Solid Edge part; units mm, degrees
sketch "Sketch1" plane through (0, 0, 0) normal (0, -1, 0) x (1, 0, 0)
  line L0 (30, 0) -> (65, 15)
  line L1 (65, 15) -> (110, 15)
  line L2 (110, 15) -> (110, 20)
  line L3 (0, 20) -> (110, 20)
  line L4 (0, 20) -> (0, 15)
  line L5 (0, 15) -> (23, 15)
  line L6 (23, 15) -> (23, 8)
  line L7 (23, 8) -> (0, 8)
  line L8 (0, 8) -> (0, 0)
  line L9 (0, 0) -> (30, 0)
  dimension "D1" = 23
extrude "Protrusion1" add sketch "Sketch1" against normal blind 50
mirror "Mirror1" about plane through (0, 25, 4) normal (-1, 0, 0) of "Protrusion1"
sketch "Sketch2" plane through (0, 0, 26) normal (0, -1, 0) x (1, 0, 0)
  line L0 (30, -16.6796) -> (43.2525, -11)
  line L1 (43.2525, -11) -> (30, -11)
  line L2 (30, -11) -> (30, -16.6796)
extrude "Cutout1" cut sketch "Sketch2" against normal through all
sketch "Sketch3" plane through (0, 25, 0) normal (0, 0, -1) x (1, 0, 0)
  circle A0 centre (-16, 21) radius 1.75
  circle A1 centre (16, 21) radius 1.75
  circle A2 centre (16, -21) radius 1.75
  circle A3 centre (-16, -21) radius 1.75
extrude "Cutout2" cut sketch "Sketch3" against normal up to next
sketch "Sketch4" plane through (0, 25, 8) normal (0, 0, 1) x (1, 0, 0)
  circle A0 centre (-16, -21) radius 3.75
  circle A1 centre (16, -21) radius 3.75
  circle A2 centre (-16, 21) radius 3.75
  circle A3 centre (16, 21) radius 3.75
extrude "Extrusionsausschnitt_4" cut sketch "Sketch4" against normal blind 4
mirror "Mirror2" about plane through (0, 0, 0) normal (1, 0, 0) of "Cutout1"
sketch "Sketch5" plane through (0, 25, 20) normal (0, 0, 1) x (1, 0, 0)
  line L0 (110, -40) -> (-110, -40)
  line L1 (-110, -40) -> (-110, 40)
  line L2 (-110, 40) -> (110, 40)
  line L3 (110, 40) -> (110, -40)
  dimension "D1" = 110
extrude "Protrusion2" add sketch "Sketch5" against normal up to vertex (5 mm away)
sketch "Sketch6" plane through (0, 25, 20) normal (0, 0, 1) x (1, 0, 0)
  circle A0 centre (-97.5, -32.5) radius 2.25
  circle A1 centre (-47.5, 32.5) radius 2.25
  circle A2 centre (-47.5, -32.5) radius 2.25
  circle A3 centre (47.5, 32.5) radius 2.25
  circle A4 centre (47.5, -32.5) radius 2.25
  circle A5 centre (97.5, -32.5) radius 2.25
  circle A6 centre (97.5, 32.5) radius 2.25
  circle A7 centre (-97.5, 32.5) radius 2.25
extrude "Cutout3" cut sketch "Sketch6" against normal up to next
chamfer "Fase_2" distance 0.5 angle 45 8 edges at (-95.25, -7.5, 15) (-95.25, 57.5, 15) (-45.25, 57.5, 15) (49.75, 57.5, 15) (99.75, 57.5, 15) (99.75, -7.5, 15) (49.75, -7.5, 15) (-45.25, -7.5, 15)
hole "Hole_1" at (-16, 46, 20) direction (0, 0, -1) diameter 10 end up to next
hole "Hole1" at (-16, 4, 20) direction (0, 0, -1) diameter 10 end up to next
hole "Hole2" at (16, 4, 20) direction (0, 0, -1) diameter 10 end up to next
hole "Hole3" at (16, 46, 20) direction (0, 0, -1) diameter 10 end up to next
properties material "Nylon, allgemein"
Input: part model. Units: mm. Frame: model coordinates. A direction names the side the tool comes from. Give positions to 0.01 mm unless a question says otherwise; leave off trailing zeros. Order: outer loops, then holes, each group sorted by start corner. A loop starts at its lowest first (then second) coordinate and runs counter-clockwise, first axis right, second up. Notation, with made-up numbers: (-16, -22.5) -> (25, -22.5) arc R13 cw to (25, -3.5) -> close; hole circle Ø5 at (80.5, 69.5). An arc over 180 degrees is marked (long way). Use one line per item in the form item = value.
1) First-contact query: pin 1 Ø4 at (x, y) = (-97.5, 57.5) entering from +Z; pin 2 Ø4.5 at (x, z) = (18.5, 10) entering from +Y; pin 3 Ø1 at (y, z) = (26, 13.5) entering from +X; pin 4 Ø2 at (y, z) = (37.5, 10.5) entering from +X. Flat tips, straight axial feed; report the tip coordinate or a pass-through.
Response values:
pin_1 = through
pin_2 = 50
pin_3 = 62.67
pin_4 = 56.83
2) Line query: probe 1 along Y at (x, z) = (16, 2.7); probe 2 along Y at (x, z) = (-47.5, 18); probe 3 along X at (y, z) = (49, 15.75). Output: solid intervals per line, ascending.
Response values:
probe_1 = 0 to 2.25, 5.75 to 44.25, 47.75 to 50
probe_2 = -15 to -9.75, -5.25 to 55.25, 59.75 to 65
probe_3 = -110 to -20, -12 to 12, 20 to 110
3) Section C-C, the plane y = 20. Return loops of the section in (x, z), and give its area (3 significant figures).
Response values:
outline = (-110, 15) -> (-65, 15) -> (-30, 0) -> (30, 0) -> (65, 15) -> (110, 15) -> (110, 20) -> (-110, 20) -> close; hole (-43.25, 15) -> (-30, 9.32) -> (-30, 15) -> close; hole (-23, 8) -> (23, 8) -> (23, 15) -> (-23, 15) -> close; hole (30, 9.32) -> (43.25, 15) -> (30, 15) -> close
area = 2,130 mm^2
4) Reachability of faces 1 (the flat face through (0.9, 50, 7.6)), 2 (the flat face through (0, 25, 8)), 3 (the cylindrical face through (-19, 50, 18)) from +Z, -Z, +X, -X, +Y, -Y: full face, straight path, thin tool, end or side. Return the list, or none.
Response values:
face_1 = -Z, +X, -X, +Y
face_2 = +Y, -Y
face_3 = +Z
5) Mould query, pull axis X, two halves, no side actions, for faces 4 (the flat face through (2, -15, 18)), 5 (the flat face through (30, 25, 12)). Classes: pulls with the +X half, pulls with the -X half, needs draft (parallel to the pull), parting line crosses it, or undercut.
Response values:
face_4 = needs draft
face_5 = undercut
6) Section B-B, the plane x = 47.5. Return loops of the section in (y, z).
Response values:
outline = (-15, 15) -> (-10.25, 15) -> (-9.75, 15.5) -> (-9.75, 20) -> (-15, 20) -> close; (-5.25, 15.5) -> (-4.75, 15) -> (0, 15) -> (0, 7.5) -> (50, 7.5) -> (50, 15) -> (54.75, 15) -> (55.25, 15.5) -> (55.25, 20) -> (-5.25, 20) -> close; (59.75, 15.5) -> (60.25, 15) -> (65, 15) -> (65, 20) -> (59.75, 20) -> close
7) Section A-A, the plane y = 57.5. Return loops of the section in (x, z).
Response values:
outline = (-110, 15) -> (-100.25, 15) -> (-99.75, 15.5) -> (-99.75, 20) -> (-110, 20) -> close; (-95.25, 15.5) -> (-94.75, 15) -> (-50.25, 15) -> (-49.75, 15.5) -> (-49.75, 20) -> (-95.25, 20) -> close; (-45.25, 15.5) -> (-44.75, 15) -> (44.75, 15) -> (45.25, 15.5) -> (45.25, 20) -> (-45.25, 20) -> close; (49.75, 15.5) -> (50.25, 15) -> (94.75, 15) -> (95.25, 15.5) -> (95.25, 20) -> (49.75, 20) -> close; (99.75, 15.5) -> (100.25, 15) -> (110, 15) -> (110, 20) -> (99.75, 20) -> close
